Geometry check sheet. Reference: the model listing, model coordinates, mm. Face numbers are marked on the shaded views. A direction names the side the tool comes from. Round coordinates to 2 decimals unless told otherwise and drop trailing zeros. Loops run counter-clockwise (first coordinate to the right, second up) from the corner with the lowest first, then second, coordinate; pieces in that order, holes last. Notation, with made-up numbers: (33, 76.25) -> (90, 76.25) arc R27 ccw to (90, 108.25) -> close; hole circle Ø8 at (46, -25). An arc over 180 degrees is marked (long way). Use a Markdown table: item, result. Add a question column.
Q1. Sectioned sample at B-B, the plane x = 23.5. Enter the section's corners in (y, z), then the cut area to 4 significant figures.
Q2. Release check for a two-part mould opening along Y. For the marked faces 4, 5 and 6 record: released by +Y, released by -Y, zero draft, split by the parting line, or undercut.
Q3. Sectioned sample at D-D, the plane x = 6.25. Enter the section's corners in (y, z).
Q4. Sectioned sample at C-C, the plane y = -14.5. Enter the section's corners in (x, z), then the cut area to 3 significant figures.
Q5. Material ranges on L1, parallel to Y at x = 15, z = -3.25; L2, parallel to Z at x = 7, y = 6.5; L3, parallel to Y at x = 20.5, z = -21, recorded low to high.
Q6. Set-up check for the marked faces 1, 2 and 3: record each of +Z, -Z, +X, -X, +Y, -Y from which the full face is reachable in a straight line by a thin tool's end or side.
Q7. Gauge pin test, flat ends, axial feed: P1, Ø3.5, axis at x = 27, z = -2, coming from the +Y side; P2, Ø4, axis at x = 1.5, y = 16.5, coming from the -Z side; P3, Ø10, axis at y = -26, z = 2.5, coming from the +X side. Record the tip position at first contact, or that the pin passes through.
Q8. Sectioned sample at A-A, the plane y = 15. Enter the section's corners in (x, z), then the cut area to 3 significant figures.
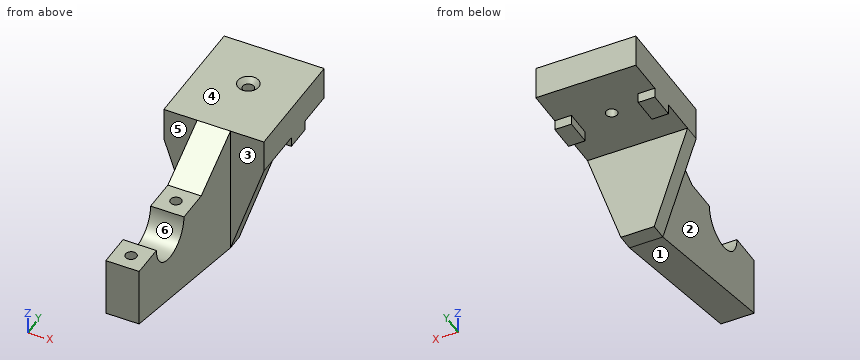
```python
from build123d import *

# Parameters (mm, degrees)
SKETCH_1_W      = 30
SKETCH_1_H      = 30
EXTRUDE_1_DEPTH = 10
EXTRUDE_2_DEPTH = 5
EXTRUDE_3_DEPTH = 5
SKETCH_6_W      = 5
SKETCH_6_H      = 8
EXTRUDE_4_DEPTH = 3


# Read off the part's stored shape, not the designer's step: 高级异型孔1, 高级异型孔2
with BuildPart() as part:
    # 草图1 → 凸台-拉伸1 (new body)
    with BuildSketch(Plane.XY):
        with Locations((15, 15)):
            Rectangle(SKETCH_1_W, SKETCH_1_H)
    extrude(amount=EXTRUDE_1_DEPTH)

    # 草图2 → 凸台-拉伸2 (add)
    with BuildSketch(Plane.XZ):
        Polygon((0, 10), (30, 10), (30, 0), (20, -30), (10, -30), (0, 0), align=None)
    extrude(amount=EXTRUDE_2_DEPTH)

    # 草图3 → 凸台-拉伸3 (add, symmetric)
    with BuildSketch(Plane(origin=(15, 0, 0), x_dir=(0, 0, -1), z_dir=(1, 0, 0))):
        with BuildLine():
            Line((0, -48), (0, -58))
            Line((0, -58), (18, -58))
            Line((18, -58), (30, -5))
            Line((30, -5), (-10, -5))
            Line((-10, -5), (0, -22))
            Line((0, -22), (0, -32))
            ThreePointArc((0, -32), (8, -40), (0, -48))
        make_face()
    extrude(amount=EXTRUDE_3_DEPTH, both=True)

    # 草图6 → 凸台-拉伸4 (add)
    with BuildSketch(Plane(origin=(0, 0, 0), x_dir=(-1, 0, 0), z_dir=(0, 0, -1))):
        with Locations((-27.5, 15)):
            Rectangle(SKETCH_6_W, SKETCH_6_H)
        with Locations((-2.5, 15)):
            Rectangle(SKETCH_6_W, SKETCH_6_H)
    extrude(amount=EXTRUDE_4_DEPTH)

    # 高级异型孔1 outline → 高级异型孔1 (revolve, cut)
    with BuildSketch(Plane(origin=(15, 15, 0), x_dir=(1, 0, 0), z_dir=(0, -1, 0))):
        Polygon((3.15, 10), (0, 10), (0, 0), (1.7, 0), (1.7, 8.55), align=None)
    revolve(axis=Axis((15, 15, 0), (0, 0, 1)), mode=Mode.SUBTRACT)

    # 高级异型孔2 outline → 高级异型孔2 (revolve, cut)
    with BuildSketch(Plane(origin=(15, -53, 0), x_dir=(1, 0, 0), z_dir=(0, -1, 0))):
        Polygon((0, -10.991420021), (1.65, -10), (1.65, 0), (0, 0), align=None)
    revolve(axis=Axis((15, -53, 0), (0, 0, 1)), mode=Mode.SUBTRACT)

    # Other 2 2 outline → Other 2 2 (revolve, cut)
    with BuildSketch(Plane(origin=(15, -27, 0), x_dir=(1, 0, 0), z_dir=(0, -1, 0))):
        Polygon((0, -10.991420021), (1.65, -10), (1.65, 0), (0, 0), align=None)
    revolve(axis=Axis((15, -27, 0), (0, 0, 1)), mode=Mode.SUBTRACT)


solid = part.part
```
Values:
| question | item | result |
|---|---|---|
| 1 | outline | (-5, -19.5) -> (0, -19.5) -> (0, 0) -> (30, 0) -> (30, 10) -> (-5, 10) -> close |
| 1 | area | 447.5 mm^2 |
| 2 | face 4 | zero draft |
| 2 | face 5 | released by -Y |
| 2 | face 6 | undercut |
| 3 | outline | (-5, -18.75) -> (0, -18.75) -> (0, 0) -> (30, 0) -> (30, 10) -> (-5, 10) -> close |
| 4 | outline | (10, -27.85) -> (20, -27.85) -> (20, 4.41) -> (10, 4.41) -> close |
| 4 | area | 323 mm^2 |
| 5 | L1 | -58 to -54.65, -51.35 to -47.31, -32.69 to -28.65, -25.35 to 0 |
| 5 | L2 | 0 to 10 |
| 5 | L3 | -5 to 0 |
| 6 | face 1 | -Z, +X, -X, -Y |
| 6 | face 2 | +Z, -Z, -X, -Y |
| 6 | face 3 | +Z, -Z, +X, -Y |
| 7 | P1 | y = 19 |
| 7 | P2 | z = -3 |
| 7 | P3 | x = 20 |
| 8 | outline | (0, -3) -> (5, -3) -> (5, 0) -> (13.3, 0) -> (13.3, 8.55) -> (11.85, 10) -> (0, 10) -> close; (16.7, 0) -> (25, 0) -> (25, -3) -> (30, -3) -> (30, 10) -> (18.15, 10) -> (16.7, 8.55) -> close |
| 8 | area | 294 mm^2 |
